Read the model definition and answer for the solid it produces. Units are mm, in the model's axes. A direction names the side the tool comes from. Round coordinates to 2 decimals unless told otherwise and drop trailing zeros. Write each loop counter-clockwise with the first axis right and the second up, starting at its lowest first coordinate (ties: lowest second). Pieces come first, ordered by that corner, then holes.
from build123d import *

# Parameters (mm, degrees)
SKETCH1_R               = 3.9
BOSS_EXTRUDE1_DEPTH     = 14
FILLET1_R               = 1
SKETCH2_R               = 0.8
CUT_EXTRUDE1_DEPTH      = 5
SKETCH3_R               = 0.8
CUT_EXTRUDE2_DEPTH      = 5
SKETCH4_W               = 2
SKETCH4_H               = 0.351785614
CUT_EXTRUDE3_DEPTH      = 5
CUT_EXTRUDE3_DEPTH_BACK = 5
SKETCH7_W               = 2
SKETCH7_H               = 1.401254955
CUT_EXTRUDE4_DEPTH      = 10
CUT_EXTRUDE4_DEPTH_BACK = 10


with BuildPart() as part:
    # Sketch1 → Boss-Extrude1 (new body)
    with BuildSketch(Plane.XY):
        Circle(SKETCH1_R)
    extrude(amount=BOSS_EXTRUDE1_DEPTH)

    # Fillet1
    fillet1_edges = [part.edges().sort_by_distance(p)[0] for p in [
        (-3.9, 0, 0),
        (-3.9, 0, 14),
    ]]
    fillet(fillet1_edges, radius=FILLET1_R)

    # Sketch2 → Cut-Extrude1 (cut)
    with BuildSketch(Plane.XY.offset(14)):
        with Locations((0, -1.5)):
            Circle(SKETCH2_R)
    extrude(amount=-CUT_EXTRUDE1_DEPTH, mode=Mode.SUBTRACT)

    # Sketch3 → Cut-Extrude2 (cut)
    with BuildSketch(Plane(origin=(0, 0, 0), x_dir=(-1, 0, 0), z_dir=(0, 0, -1))):
        with Locations((0, -1.5)):
            Circle(SKETCH3_R)
    extrude(amount=-CUT_EXTRUDE2_DEPTH, mode=Mode.SUBTRACT)

    # Sketch4 → Cut-Extrude3 (cut, two sides)
    with BuildSketch(Plane(origin=(0, 0, 0), x_dir=(0, 0, -1), z_dir=(1, 0, 0))) as cut_extrude3_sk:
        with Locations((-3.521882016, 3.724107193)):
            Rectangle(SKETCH4_W, SKETCH4_H)
    extrude(amount=CUT_EXTRUDE3_DEPTH, mode=Mode.SUBTRACT)
    extrude(cut_extrude3_sk.sketch, amount=-CUT_EXTRUDE3_DEPTH_BACK, mode=Mode.SUBTRACT)

    # Sketch7 → Cut-Extrude4 (cut, two sides)
    with BuildSketch(Plane(origin=(0, 0, 0), x_dir=(0, 0, -1), z_dir=(1, 0, 0))) as cut_extrude4_sk:
        with Locations((-11.03673309, 4.248841864)):
            Rectangle(SKETCH7_W, SKETCH7_H)
    extrude(amount=CUT_EXTRUDE4_DEPTH, mode=Mode.SUBTRACT)
    extrude(cut_extrude4_sk.sketch, amount=-CUT_EXTRUDE4_DEPTH_BACK, mode=Mode.SUBTRACT)


solid = part.part
Q1. Determine the mould class of faces 1 (the cylindrical face through (-0.845, -3.807, 6.916)), 2 (the flat face through (0, -1, 9)), 3 (the flat face through (0, 3.548, 11)), 4 (the flat face through (0, -1, 5)) for opening direction X: pulls with the +X half, pulls with the -X half, needs draft (parallel to the pull), parting line crosses it, or undercut.
Verdict:
face 1: parting line crosses it
face 2: undercut
face 3: needs draft
face 4: undercut
Q2. Section A-A (z = 12.75) is taken. Determine the outline of the cut face in (x, y).
Verdict:
outline: circle Ø7.8 at (0, 0); hole circle Ø1.6 at (0, -1.5)
Q3. Straight lines are drawn through the part: probe 1 along Y at (x, z) = (0, 3.3); probe 2 along Y at (x, z) = (0, 12.95); probe 3 along Z at (x, y) = (0, -2.25). For each, find the intervals that lie inside material, in ascending order.
Verdict:
probe 1: y = -3.9 to -2.3, -0.7 to 3.55
probe 2: y = -3.9 to -2.3, -0.7 to 3.9
probe 3: z = 5 to 9
Q4. Flat-ended cylindrical pins translate along their axes: pin 1 Ø2 at (x, z) = (-2.5, 11.5) entering from -Y; pin 2 Ø2 at (y, z) = (-1.5, 8.5) entering from +X; pin 3 Ø0.6 at (x, z) = (0, 11) entering from +Y. Find the tip coordinate at first contact, or state that the pin passes through.
Verdict:
pin 1: stops at y = -3.6
pin 2: stops at x = 3.87
pin 3: stops at y = 3.55
Q5. Which of the six approach directions +Z, -Z, +X, -X, +Y, -Y give full straight-line access (tool end or side, diameter ignored) to faces 5 (the flat face through (0, 0, 0)), 6 (the flat face through (0, 3.548, 4)), 7 (the cylindrical face through (-0.17, -2.28, 11.54)), 8 (the cylindrical face through (0.17, -2.28, 2.46))?
Verdict:
face 5: -Z, +X, -X, +Y, -Y
face 6: +X, -X, +Y
face 7: +Z
face 8: -Z
Q6. Section B-B (x = 0) is taken. Determine the outline of the cut face in (y, z).
Verdict:
outline: (-3.9, 1) arc R1 ccw to (-2.9, 0) - (-2.3, 0) - (-2.3, 5) - (-0.7, 5) - (-0.7, 0) - (2.9, 0) arc R1 ccw to (3.9, 1) - (3.9, 2.52) - (3.55, 2.52) - (3.55, 4.52) - (3.9, 4.52) - (3.9, 10.04) - (3.55, 10.04) - (3.55, 12.04) - (3.9, 12.04) - (3.9, 13) arc R1 ccw to (2.9, 14) - (-0.7, 14) - (-0.7, 9) - (-2.3, 9) - (-2.3, 14) - (-2.9, 14) arc R1 ccw to (-3.9, 13) - close
